Geometry: see drawing. Coordinates: mm, zero at the bounding-box minimum. Give positions to 0.01 mm unless a question says otherwise; leave off trailing zeros. Order: outer loops, then holes, each group sorted by start corner. A loop starts at its lowest first (then second) coordinate and runs counter-clockwise, first axis right, second up. Notation, with made-up numbers: (26.5, 67.5) -> (80.5, 67.5) arc R22 ccw to (80.5, 82.5) -> close; hole circle Ø2 at (57.5, -8.75). An arc over 180 degrees is marked (long way). Use one line per item in the form item = value. Start each with the question number.
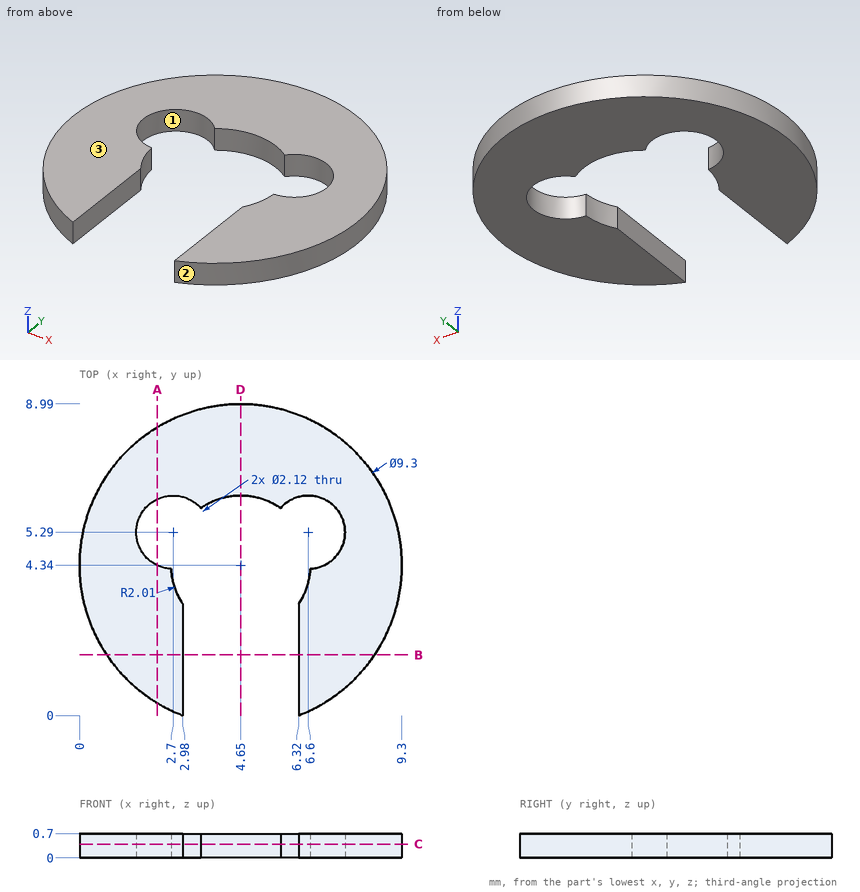
1) Cut plane B-B, the plane y = 1.75. Return the cut outline in (x, z).
2) Cut plane A-A, the plane x = 2.25. Return the cut outline in (y, z).
3) Material intervals for probe 1 along X at (y, z) = (4.5, 0.45); probe 2 along Y at (x, z) = (2, 0.65) (1 decimal); probe 3 along X at (y, z) = (4.75, 0.65), sorted ascending.
4) Pin query (flat end, axial travel): pin 1 (3 mm diameter, centred on x = 6.6, y = 5.29, fed in from +Z). Return the tip coordinate at first contact, or that it passes through.
5) Cut plane C-C, the plane z = 0.4. Return the cut outline in (x, y).
6) Cut plane D-D, the plane x = 4.65. Return the cut outline in (y, z).
7) Draft query along X for the marked faces 1, 2 and 3. Return one class per face: +X half, -X half, draft (parallel to the pull), parting line (faces both ways), or undercut.
Output values:
q1.outline = (0.79, 0) -> (2.98, 0) -> (2.98, 0.7) -> (0.79, 0.7) -> close; (6.32, 0) -> (8.51, 0) -> (8.51, 0.7) -> (6.32, 0.7) -> close
q2.outline = (0.36, 0) -> (4.33, 0) -> (4.33, 0.7) -> (0.36, 0.7) -> close; (6.25, 0) -> (8.32, 0) -> (8.32, 0.7) -> (6.25, 0.7) -> close
q3.probe_1 = 0 to 1.99, 7.31 to 9.3
q3.probe_2 = 0.5 to 4.5, 6.1 to 8.2
q3.probe_3 = 0.02 to 1.79, 7.51 to 9.28
q4.pin_1 = 0.7
q5.outline = (2.64, 4.23) arc R1.06 cw (long way) to (3.5, 5.99) arc R2.01 cw to (5.8, 5.99) arc R1.06 cw (long way) to (6.66, 4.23) arc R2.01 cw to (6.32, 3.22) -> (6.32, 0) arc R4.65 ccw (long way) to (2.98, 0) -> (2.98, 3.22) arc R2.01 cw to start
q6.outline = (6.35, 0) -> (8.99, 0) -> (8.99, 0.7) -> (6.35, 0.7) -> close
q7.face_1 = undercut
q7.face_2 = parting line
q7.face_3 = draft
